The listing builds one solid part. Answer for the finished solid, in the listing's coordinates (mm). Give positions to 0.01 mm unless a question says otherwise; leave off trailing zeros. Order: outer loops, then holes, each group sorted by start corner. A loop starts at its lowest first (then second) coordinate and runs counter-clockwise, first axis right, second up.
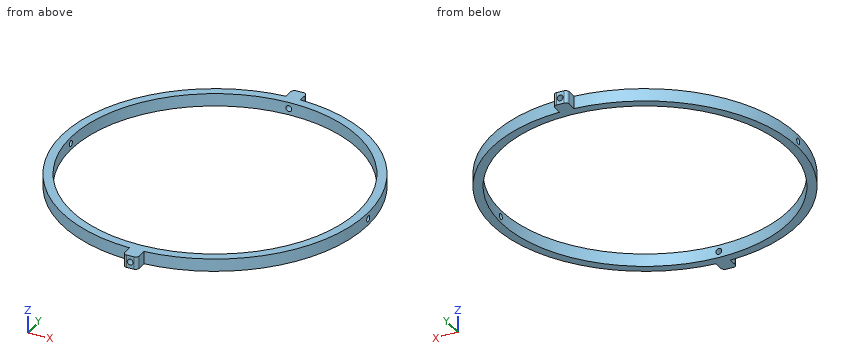
```python
from build123d import *

# Parameters (mm, degrees)
SKETCH074_R          = 85
SKETCH074_R_2        = 80
SKETCH074_W          = 8
SKETCH074_H          = 12
PAD006_DEPTH         = 3.5
PAD007_DEPTH         = 3.5
SKETCH076_R          = 1.65
POCKET004_DEPTH      = 85.001
POCKET004_DEPTH_BACK = 85.001
SKETCH075_R          = 1.65
POCKET005_DEPTH      = 92.001
POCKET005_DEPTH_BACK = 92.001
FILLET001_R          = 2


with BuildPart() as part:
    # Sketch074 → Pad006 (new body, symmetric)
    with BuildSketch(Plane.XY):
        Circle(SKETCH074_R)
        Circle(SKETCH074_R_2, mode=Mode.SUBTRACT)
        with Locations((0, 86)):
            Rectangle(SKETCH074_W, SKETCH074_H)
        with Locations((0, -86)):
            Rectangle(SKETCH074_W, SKETCH074_H)
    extrude(amount=PAD006_DEPTH, both=True)

    # Sketch074 → Pad007 (join, symmetric)
    with BuildSketch(Plane.XY):
        Circle(SKETCH074_R)
        Circle(SKETCH074_R_2, mode=Mode.SUBTRACT)
        with Locations((0, 86)):
            Rectangle(SKETCH074_W, SKETCH074_H)
        with Locations((0, -86)):
            Rectangle(SKETCH074_W, SKETCH074_H)
    extrude(amount=PAD007_DEPTH, both=True)

    # Sketch076 → Pocket004 (cut, two sides)
    with BuildSketch(Plane.YZ) as pocket004_sk:
        Circle(SKETCH076_R)
    extrude(amount=-POCKET004_DEPTH, mode=Mode.SUBTRACT)
    extrude(pocket004_sk.sketch, amount=POCKET004_DEPTH_BACK, mode=Mode.SUBTRACT)

    # Sketch075 → Pocket005 (cut, two sides)
    with BuildSketch(Plane.XZ) as pocket005_sk:
        Circle(SKETCH075_R)
    extrude(amount=-POCKET005_DEPTH, mode=Mode.SUBTRACT)
    extrude(pocket005_sk.sketch, amount=POCKET005_DEPTH_BACK, mode=Mode.SUBTRACT)

    # Fillet001
    fillet001_edges = [part.edges().sort_by_distance(p)[0] for p in [
        (4, -92, 0),
        (-4, -92, 0),
        (-4, 92, 0),
        (4, 92, 0),
    ]]
    fillet(fillet001_edges, radius=FILLET001_R)


solid = part.part
```
1) Straight lines are drawn through the part: probe 1 along Z at (x, y) = (-83.25, 0); probe 2 along X at (y, z) = (1, -2.5); probe 3 along Y at (x, z) = (-55, 2.5). For each, find the intervals that lie inside material, in ascending order.
Geometry says:
probe 1: z = -3.5 to -1.65, 1.65 to 3.5
probe 2: x = -84.99 to -79.99, 79.99 to 84.99
probe 3: y = -64.81 to -58.09, 58.09 to 64.81
2) Find section C-C (z = 0). Write down the section's boundary in (x, y).
Geometry says:
outline: (-84.98, -1.65) arc R85 ccw to (-4, -84.91) - (-4, -90) arc R2 ccw to (-2, -92) - (-1.65, -92) - (-1.65, -79.98) arc R80 cw to (-79.98, -1.65) - close; (-84.98, 1.65) - (-79.98, 1.65) arc R80 cw to (-1.65, 79.98) - (-1.65, 92) - (-2, 92) arc R2 ccw to (-4, 90) - (-4, 84.91) arc R85 ccw to start; (1.65, -92) - (2, -92) arc R2 ccw to (4, -90) - (4, -84.91) arc R85 ccw to (84.98, -1.65) - (79.98, -1.65) arc R80 cw to (1.65, -79.98) - close; (1.65, 79.98) arc R80 cw to (79.98, 1.65) - (84.98, 1.65) arc R85 ccw to (4, 84.91) - (4, 90) arc R2 ccw to (2, 92) - (1.65, 92) - close
3) Find section B-B (x = 41). Write down the section's boundary in (y, z).
Geometry says:
outline: (-74.46, -3.5) - (-68.69, -3.5) - (-68.69, 3.5) - (-74.46, 3.5) - close; (68.69, -3.5) - (74.46, -3.5) - (74.46, 3.5) - (68.69, 3.5) - close
4) Find section A-A (y = 13). Write down the section's boundary in (x, z), then the cut area to 3 significant figures.
Geometry says:
outline: (-84, -3.5) - (-78.94, -3.5) - (-78.94, 3.5) - (-84, 3.5) - close; (78.94, -3.5) - (84, -3.5) - (84, 3.5) - (78.94, 3.5) - close
area: 70.9 mm2
5) Given P1, Ø2, axis at x = -6, z = -2.5, coming from the +Y side; P2, Ø3, axis at y = 0, z = 0, coming from the +X side; P3, Ø2.5, axis at y = -87.5, z = 1, coming from the +X side; P4, Ø1.5, axis at x = -13.5, z = -2, coming from the -Y side, each flat-ended and moving along its own axis, determine where each tip first touches the part or whether it passes through.
Geometry says:
P1: stops at y = 84.85
P2: passes through
P3: stops at x = 4
P4: stops at y = -84.04
